```python
from build123d import *

# Parameters (mm, degrees)
BOSS_EXTRUDE1_DEPTH = 38.1
SKETCH3_R           = 3.302
CUT_EXTRUDE1_DEPTH  = 23.225
FILLET1_R           = 6.35
FILLET2_R           = 12.7


with BuildPart() as part:
    # Sketch1 → Boss-Extrude1 (new body)
    with BuildSketch(Plane(origin=(0, 0, 0), x_dir=(0, 0, -1), z_dir=(1, 0, 0))):
        Polygon((0, 0), (-22.225, 0), (-22.225, 12.7), (-3.175, 12.7), (-3.175, 31.75), (0, 31.75), align=None)
    extrude(amount=BOSS_EXTRUDE1_DEPTH)

    # Sketch3 → Cut-Extrude1 (cut, through all)
    with BuildSketch(Plane(origin=(0, 0, 0), x_dir=(-1, 0, 0), z_dir=(0, 0, -1))):
        with Locations((-19.05, 24.13)):
            Circle(SKETCH3_R)
    extrude(amount=-CUT_EXTRUDE1_DEPTH, mode=Mode.SUBTRACT)

    # Fillet1
    fillet1_edges = [part.edges().sort_by_distance(p)[0] for p in [
        (38.1, 6.35, 22.225),
        (0, 6.35, 22.225),
    ]]
    fillet(fillet1_edges, radius=FILLET1_R)

    # Fillet2
    fillet2_edges = [part.edges().sort_by_distance(p)[0] for p in [
        (0, 31.75, 1.5875),
        (38.1, 31.75, 1.5875),
    ]]
    fillet(fillet2_edges, radius=FILLET2_R)


solid = part.part
```
Could you check a few things on this model? Use its own coordinates, in mm. A direction names the side the tool comes from. Round coordinates to 2 decimals unless told otherwise and drop trailing zeros. Loops run counter-clockwise (first coordinate to the right, second up) from the corner with the lowest first, then second, coordinate; pieces in that order, holes last. Notation, with made-up numbers: M 25.5,-8 L 54.5,-8 A8 ccw 54.5,7 Z; hole C -23,46 d11. An arc over 180 degrees is marked long. Write item = value, one per line.
1. I want a section at B-B, the plane y = 24.13. Write out the boundary of the cut face in (x, z) (3 decimals), and give its area (3 significant figures).
Results below:
outline = M 1.06,0 L 15.748,0 L 15.748,3.175 L 1.06,3.175 Z; M 22.352,0 L 37.04,0 L 37.04,3.175 L 22.352,3.175 Z
area = 93.3 mm²
2. Will these pins go through, and if not, where does the flat tip stop? P1, Ø15, axis at x = 23.5, y = 24.5, coming from the +Z side (3 decimals); P2, Ø5, axis at x = 25, z = 16.5, coming from the +Y side.
Results below:
P1 = 3.175
P2 = 12.7
3. Thinking about a two-plate mould opening in X: for faces 1 (the face through (19.5, 27.4, 1.6)), 2 (the face through (0, 8, 8)), 3 (the face through (19, 31.75, 2)), which applies, +X half, -X half, draft (parallel to the pull), parting line (faces both ways), or undercut?
Results below:
face_1 = undercut
face_2 = -X half
face_3 = draft
4. I want a section at D-D, the plane y = 7. Write out the boundary of the cut face in (x, z) (3 decimals).
Results below:
outline = M 0,0 L 38.1,0 L 38.1,15.875 A6.35 ccw 31.75,22.225 L 6.35,22.225 A6.35 ccw 0,15.875 Z
5. Which directions (+Z, -Z, +X, -X, +Y, -Y) give clear straight access to the entire face, cutting with the end or side of a thin tool? Please do faces 4 (the face through (34.48, 27.93, 1.57)), 5 (the face through (19, 12.7, 13)).
Results below:
face_4 = +Z, -Z, +X, +Y
face_5 = +Z, +X, -X, +Y
6. I want a section at A-A, the plane x = 19.05. Write out the boundary of the cut face in (y, z) (3 decimals), and give its area (3 significant figures).
Results below:
outline = M 0,0 L 20.828,0 L 20.828,3.175 L 12.7,3.175 L 12.7,22.225 L 0,22.225 Z; M 27.432,0 L 31.75,0 L 31.75,3.175 L 27.432,3.175 Z
area = 322 mm²
7. I want a section at C-C, the plane z = 13.25. Write out the boundary of the cut face in (x, y), and give its area (3 significant figures).
Results below:
outline = M 0,0 L 38.1,0 L 38.1,12.7 L 0,12.7 Z
area = 484 mm²
8. I need wall thicknesses on probe 1 along Y at (x, z) = (19.05, 1.9); probe 2 along Y at (x, z) = (16.5, 15.25); probe 3 along Z at (x, y) = (22.5, 17) (3 decimals). Which ranges of each line are inside material? Lowest first, please.
Results below:
probe_1 = 0 to 20.83, 27.43 to 31.75
probe_2 = 0 to 12.7
probe_3 = 0 to 3.175
